Model file for the job. Use its own axes, mm. Face numbers are marked on the shaded views. A direction names the side the tool comes from. Coordinates: 2 decimals unless noted, no trailing zeros. Write each loop counter-clockwise with the first axis right and the second up, starting at its lowest first coordinate (ties: lowest second). Pieces come first, ordered by that corner, then holes. Notation, with made-up numbers: M 78.5,-7.5 L 104.5,-7.5 A23 cw 104.5,15.5 Z; hole C -26,55 d6. An arc over 180 degrees is marked long. Use CSV: the item, a comma, the result in double quotes. Start each with the question number.
from build123d import *

# Parameters (mm, degrees)
EXTRUDE_1_DEPTH          = 473.5
CUT_EXTRUDE_1_DEPTH      = 505.35230742
CUT_EXTRUDE_1_DEPTH_BACK = 505.35230742
SKETCH_2_R               = 2.5


with BuildPart() as part:
    # Эскиз1 → Бобышка-Вытянуть1 (new, symmetric)
    with BuildSketch(Plane.XY):
        with BuildLine():
            Line((71.5, 0), (-71.5, 0))
            ThreePointArc((-71.5, 0), (-78.571067812, 2.928932188), (-81.5, 10))
            Line((-81.5, 10), (-81.5, 60))
            Line((-81.5, 60), (-76.5, 60))
            Line((-76.5, 60), (-76.5, 10))
            ThreePointArc((-76.5, 10), (-75.035533906, 6.464466094), (-71.5, 5))
            Line((-71.5, 5), (71.5, 5))
            ThreePointArc((71.5, 5), (75.035533906, 6.464466094), (76.5, 10))
            Line((76.5, 10), (76.5, 60))
            Line((76.5, 60), (81.5, 60))
            Line((81.5, 60), (81.5, 10))
            ThreePointArc((81.5, 10), (78.571067812, 2.928932188), (71.5, 0))
        make_face()
    extrude(amount=EXTRUDE_1_DEPTH, both=True)

    # Эскиз2 → Вырез-Вытянуть1 (cut, two sides: drawn at the far end of the back side and taken through both)
    with BuildSketch(Plane.ZY.offset(81.5).offset(-CUT_EXTRUDE_1_DEPTH_BACK)):
        with Locations((-433.5, 24.9115)):
            Circle(SKETCH_2_R)
        with Locations((-293.5, 24.9115)):
            Circle(SKETCH_2_R)
    extrude(amount=CUT_EXTRUDE_1_DEPTH + CUT_EXTRUDE_1_DEPTH_BACK, mode=Mode.SUBTRACT)


solid = part.part
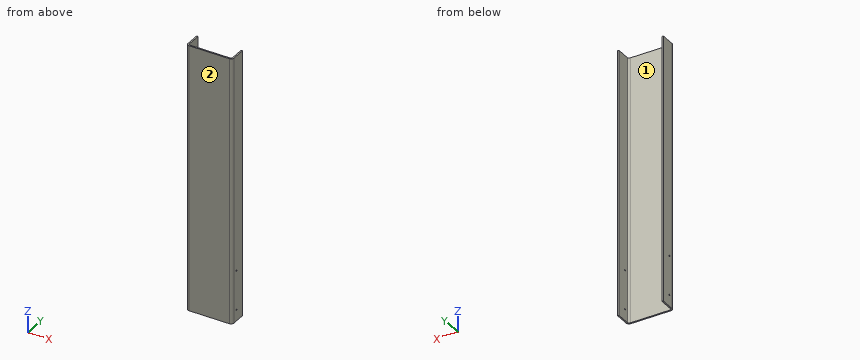
1) Drop a flat-ended pin along its axis: P1, Ø2, axis at x = 64.5, z = -120.5, coming from the +Y side. Give the stop position or say it passes through.
2) Wall check: L1, parallel to X at y = 16.5, z = 324.5; L2, parallel to Y at x = -62.5, z = 264; L3, parallel to X at y = 8, z = -11.5. Give the ranges that are in metal, low to high. Write a range as [from, to].
3) Band-saw the part on A-A on y = 45.5. List the corners of the cut face in (x, z).
4) Band-saw the part on B-B on z = -208.5. List the corners of the cut face in (x, y).
5) Tool access for the marked faces 1 and 2: list every direction of +Z, -Z, +X, -X, +Y, -Y with a clear straight run to the whole face (end or side of a thin tool).
6) Band-saw the part on C-C on x = -29. List the corners of the cut face in (y, z), then the cut area to 4 significant figures.
Findings below:
1,P1,"stops at y = 5"
2,L1,"x = [-81.5, -76.5], [76.5, 81.5]"
2,L2,"y = [0, 5]"
2,L3,"x = [-81.3, -76.08], [76.08, 81.3]"
3,outline,"M -81.5,-473.5 L -76.5,-473.5 L -76.5,473.5 L -81.5,473.5 Z; M 76.5,-473.5 L 81.5,-473.5 L 81.5,473.5 L 76.5,473.5 Z"
4,outline,"M -81.5,10 A10 ccw -71.5,0 L 71.5,0 A10 ccw 81.5,10 L 81.5,60 L 76.5,60 L 76.5,10 A5 cw 71.5,5 L -71.5,5 A5 cw -76.5,10 L -76.5,60 L -81.5,60 Z"
5,face 1,"+Z, -Z, +Y"
5,face 2,"+Z, -Z, +X, -X, -Y"
6,outline,"M 0,-473.5 L 5,-473.5 L 5,473.5 L 0,473.5 Z"
6,area,"4,735 mm2"
